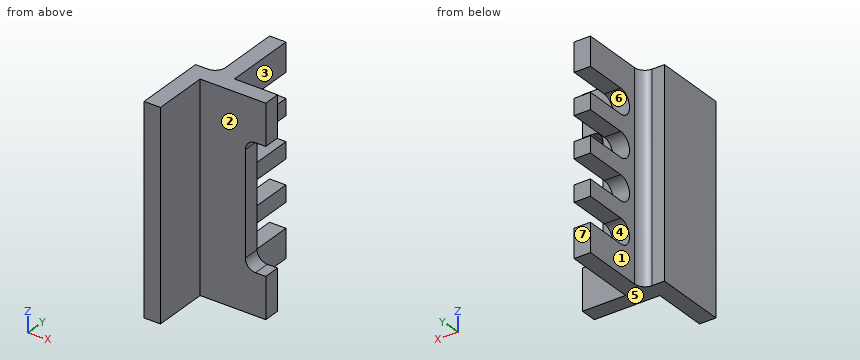
from build123d import *

# Parameters (mm, degrees)
BOSS_EXTRUDE1_DEPTH = 100
SKETCH3_W           = 10
SKETCH3_H           = 60
CUT_EXTRUDE1_DEPTH  = 8
CUT_EXTRUDE2_DEPTH  = 8
LPATTERN1_COUNT     = 4
LPATTERN1_PITCH     = 20
FILLET1_R           = 5


with BuildPart() as part:
    # Sketch2 → Boss-Extrude1 (new body)
    with BuildSketch(Plane.XY):
        Polygon((0, 0), (0, -35), (8, -35), (8, -8), (40, -8), (40, 0), (19, 0), (19, 35), (11, 35), (11, 0), align=None)
    extrude(amount=BOSS_EXTRUDE1_DEPTH)

    # Sketch3 → Cut-Extrude1 (cut)
    with BuildSketch(Plane(origin=(0, 0, 0), x_dir=(1, 0, 0), z_dir=(0, 1, 0))):
        with Locations((35, -50)):
            Rectangle(SKETCH3_W, SKETCH3_H)
    extrude(amount=-CUT_EXTRUDE1_DEPTH, mode=Mode.SUBTRACT)

    # Sketch4 → Cut-Extrude2 (cut)
    with BuildSketch(Plane(origin=(19, 0, 0), x_dir=(0, 0, -1), z_dir=(1, 0, 0))):
        with BuildLine():
            Line((-86, 35), (-86, 14.440154261))
            ThreePointArc((-86, 14.440154261), (-80, 8.440154261), (-74, 14.440154261))
            Line((-74, 14.440154261), (-74, 35))
            Line((-74, 35), (-86, 35))
        make_face()
    cut_extrude2 = extrude(amount=-CUT_EXTRUDE2_DEPTH, mode=Mode.SUBTRACT)

    # LPattern1: Cut-Extrude2 ×4
    with Locations(*[(0, 0, -i * LPATTERN1_PITCH) for i in range(1, LPATTERN1_COUNT)]):
        add(cut_extrude2, mode=Mode.SUBTRACT)

    # Fillet1
    fillet1_edges = [part.edges().sort_by_distance(p)[0] for p in [
        (11, 0, 50),
        (30, -4, 80),
        (30, -4, 20),
    ]]
    fillet(fillet1_edges, radius=FILLET1_R)


solid = part.part
Could you check a few things on this model? Use its own coordinates, in mm. Face numbers are marked on the shaded views. A direction names the side the tool comes from. Give positions to 0.01 mm unless a question says otherwise; leave off trailing zeros. Loops run counter-clockwise (first coordinate to the right, second up) from the corner with the lowest first, then second, coordinate; pieces in that order, holes last. Notation, with made-up numbers: (22.5, 74) -> (70.5, 74) arc R38 cw to (70.5, 113) -> close; hole circle Ø5 at (4.5, 17.5). An arc over 180 degrees is marked (long way). Answer as CSV lines item,"result". Start each with the question number.
(1) If we section it at B-B on x = 17: Write out the boundary of the cut face in (y, z).
(2) I need wall thicknesses on probe 1 along Z at (x, y) = (12.5, 17.5); probe 2 along X at (y, z) = (-19, 93); probe 3 along Y at (x, z) = (25.5, 48.5). Which ranges of each line are inside material? Lowest first, please.
(3) Which directions (+Z, -Z, +X, -X, +Y, -Y) give clear straight access to the entire face, cutting with the end or side of a thin tool? Please do the marked faces 1, 2 and 3.
(4) I'm going to push flat-ended pins straight in: pin 1 Ø2.5 at (y, z) = (-4, 47) entering from +X; pin 2 Ø4 at (y, z) = (24, 51) entering from -X; pin 3 Ø2 at (y, z) = (25.5, 53.5) entering from +X. Where does each tip first touch, or does it pass through?
(5) If we section it at D-D on z = 50: Write out the boundary of the cut face in (x, y).
(6) We'd pull the mould along Z, two halves only. Please class the marked faces 4, 5, 6 and 7: released by +Z, released by -Z, zero draft, split by the parting line, or undercut.
(7) If we section it at C-C on y = -24: Write out the boundary of the cut face in (x, z).
(8) If we section it at A-A on z = 60: Write out the boundary of the cut face in (x, y), then the cut area to 3 significant figures.
Computed:
1,outline,"(-8, 0) -> (35, 0) -> (35, 14) -> (14.44, 14) arc R6 cw to (14.44, 26) -> (35, 26) -> (35, 34) -> (14.44, 34) arc R6 cw to (14.44, 46) -> (35, 46) -> (35, 54) -> (14.44, 54) arc R6 cw to (14.44, 66) -> (35, 66) -> (35, 74) -> (14.44, 74) arc R6 cw to (14.44, 86) -> (35, 86) -> (35, 100) -> (-8, 100) -> close"
2,probe 1,"z = 0 to 14, 26 to 34, 46 to 54, 66 to 74, 86 to 100"
2,probe 2,"x = 0 to 8"
2,probe 3,"y = -8 to 0"
3,face 1,"+Z, -Z, -X, +Y"
3,face 2,"+Z, -Z, +X, -Y"
3,face 3,"+Z, -Z, +X, +Y"
4,pin 1,"stops at x = 30"
4,pin 2,"stops at x = 11"
4,pin 3,"stops at x = 19"
5,outline,"(0, -35) -> (8, -35) -> (8, -8) -> (30, -8) -> (30, 0) -> (19, 0) -> (19, 35) -> (11, 35) -> (11, 5) arc R5 cw to (6, 0) -> (0, 0) -> close"
6,face 4,"undercut"
6,face 5,"released by -Z"
6,face 6,"undercut"
6,face 7,"zero draft"
7,outline,"(0, 0) -> (8, 0) -> (8, 100) -> (0, 100) -> close"
8,outline,"(0, -35) -> (8, -35) -> (8, -8) -> (30, -8) -> (30, 0) -> (19, 0) -> (19, 8.44) -> (11, 8.44) -> (11, 5) arc R5 cw to (6, 0) -> (0, 0) -> close"
8,area,"529 mm2"
